Design review of the part built by this model. Coordinates are the model's own, in mm. Round coordinates to 2 decimals unless told otherwise and drop trailing zeros. Order: outer loops, then holes, each group sorted by start corner. A loop starts at its lowest first (then second) coordinate and runs counter-clockwise, first axis right, second up. Notation, with made-up numbers: (-17.75, 55) - (-3.75, 55) arc R24 cw to (-3.75, 67) - close; hole circle Ø3 at (-24.75, 40). An arc over 180 degrees is marked (long way). Write item = value, one per line.
Autodesk Inventor part; units mm, degrees
ref_plane "YZ Plane" through (0, 0, 0) normal (1, 0, 0) x (0, 1, 0)
ref_plane "XZ Plane" through (0, 0, 0) normal (0, 1, 0) x (-1, 0, 0)
ref_plane "XY Plane" through (0, 0, 0) normal (0, 0, 1) x (1, 0, 0)
sketch "Sketch1" plane through (0, 0, 0) normal (1, 0, 0) x (0, 1, 0)
  line L0 (0, 0) -> (3.2512, 0)
  line L1 (3.2512, 0) -> (3.2512, -25.4)
  line L2 (3.2512, -25.4) -> (0, -25.4)
  line L3 (0, -25.4) -> (0, 0)
  dimension "d0" = 3.2512
  dimension "d1" = 25.4
extrude "Extrusion1" add sketch "Sketch1" along normal blind 381
sketch "Sketch2" plane through (0, 3.2512, 0) normal (0, 1, 0) x (1, 0, 0)
  line L0 (0, 25.4) -> (0, 0)
  line L1 (0, 12.7) -> (85.4474, 12.7) construction
  circle A0 centre (10.8949, 12.7) radius 3.175
  line L2 (0, 0) -> (381, 0)
  line L3 (190.5, 0) -> (190.5, 15.076) construction
  line L4 (381, 12.7) -> (295.5526, 12.7) construction
  circle A1 centre (370.1051, 12.7) radius 3.175
  dimension "d4" = 6.35
  dimension "d5" = 179.6051
extrude "Extrusion2" cut sketch "Sketch2" against normal blind 381
properties part number "Long support flat"
Item 1: Insertion check: P1, Ø8.5, axis at x = 370.11, z = -12.7, coming from the +Y side; P2, Ø4, axis at x = 10.89, z = -12.7, coming from the -Y side. Each pin has a flat end and moves straight along its axis. Give the tip position at first contact, or say it passes through.
Data:
P1 = 3.25
P2 = through
Item 2: For line 1 along X through (y, z) = (2.1, -12.7); line 2 along X through (y, z) = (0.5, -11), list the stretches that pass through material, from the lowest coordinate up. Write a range as [from, to].
Data:
line_1 = [0, 7.72], [14.07, 366.93], [373.28, 381]
line_2 = [0, 8.21], [13.58, 367.42], [372.79, 381]
Item 3: The part is to be moulded in two halves that separate along X. For faces 1 (the face through (8.375, 1.648, -10.768)), 2 (the face through (188, 3.251, -13)), say which applies: +X half, -X half, draft (parallel to the pull), parting line (faces both ways), or undercut.
Data:
face_1 = undercut
face_2 = draft
Item 4: Take a section at A-A, the plane z = -12.7. State the section outline as (x, y) points.
Data:
outline = (0, 0) - (7.72, 0) - (7.72, 3.25) - (0, 3.25) - close; (14.07, 0) - (366.93, 0) - (366.93, 3.25) - (14.07, 3.25) - close; (373.28, 0) - (381, 0) - (381, 3.25) - (373.28, 3.25) - close
